Geometry check sheet. Reference: the model listing, model coordinates, mm. A direction names the side the tool comes from. Give positions to 0.01 mm unless a question says otherwise; leave off trailing zeros. Loops run counter-clockwise (first coordinate to the right, second up) from the corner with the lowest first, then second, coordinate; pieces in that order, holes last. Notation, with made-up numbers: (-38, -33.5) - (2, -33.5) arc R21 cw to (2, 0.5) - close; hole circle Ø1 at (71.25, -31). An arc over 180 degrees is marked (long way). Use a Markdown table: item, result. Add a question column.
1. Set-up check for faces 1 (the flat face through (0, -21.59, 0)), 2 (the flat face through (-1, 0, -20.32)), 3 (the flat face through (20.32, 0, 23)), 4 (the flat face through (-1.905, 0, 23)): record each of +Z, -Z, +X, -X, +Y, -Y from which the full face is reachable in a straight line by a thin tool's end or side.
2. Cross-section at A-A on x = 4. Enter the section's corners in (y, z), and give its area (3 significant figures).
3. Draft check along Z on faces 5 (the flat face through (0, -25.4, 0)), 6 (the flat face through (0, 0, -25.4)), 7 (the flat face through (1, 0, 20.32)). Enter one of: pulls with the +Z half, pulls with the -Z half, needs draft (parallel to the pull), parting line crosses it, or undercut.
4. Cross-section at D-D on z = -22. Enter the section's corners in (x, y) (3 decimals), and give its area (3 significant figures).
5. Material ranges on L1, parallel to Y at x = -13.5, z = 2; L2, parallel to X at y = -17.5, z = -23 (3 decimals); L3, parallel to Z at x = 1.5, y = 5, recorded low to high.
6. Cross-section at B-B on y = -11.5. Count the separate pieces of the cut face and the enclosed holes in it, and give its area (3 significant figures).
7. Cross-section at C-C on z = 17. Enter the section's corners in (x, y).
8. Depth check by flat-ended pin: P1, Ø6, axis at x = 5.5, y = 4.5, coming from the +Z side. Enter the tip coordinate at first touch or a pass-through.
from build123d import *

# Parameters (mm, degrees)
SKETCH1_W           = 5.08
SKETCH1_H           = 5.08
BOSS_EXTRUDE1_DEPTH = 21.59
LPATTERN2_COUNT     = 3
LPATTERN2_PITCH     = 22.86
LPATTERN3_COUNT     = 2
LPATTERN3_PITCH     = 23.495
LPATTERN4_COUNT     = 2
LPATTERN4_PITCH     = 23.495
SKETCH2_W           = 50.8
SKETCH2_H           = 50.8
BOSS_EXTRUDE3_DEPTH = 3.81
SKETCH3_W           = 50.8
SKETCH3_H           = 50.8
BOSS_EXTRUDE4_DEPTH = 3.81


with BuildPart() as part:
    # Sketch1 → Boss-Extrude1 (new body, symmetric)
    with BuildSketch(Plane(origin=(0, 0, 0), x_dir=(1, 0, 0), z_dir=(0, 1, 0))):
        with Locations((-22.86, -22.86)):
            Rectangle(SKETCH1_W, SKETCH1_H)
    extrude(amount=BOSS_EXTRUDE1_DEPTH, both=True)


with BuildPart() as lpattern2_1:
    # LPattern2: pattern copy
    add(part.part.moved(Location(Vector(0, 0, -1) * (1 * LPATTERN2_PITCH))))


with BuildPart() as lpattern2_2:
    # LPattern2: pattern copy
    add(part.part.moved(Location(Vector(0, 0, -1) * (2 * LPATTERN2_PITCH))))


with BuildPart() as body_4:
    # Mirror1: mirrored copy
    add(lpattern2_2.part.mirror(Plane(origin=(0, 0, 0), x_dir=(0, 0, 1), z_dir=(1, 0, 0))))


with BuildPart() as body_5:
    # Mirror1 2: mirrored copy
    add(lpattern2_1.part.mirror(Plane(origin=(0, 0, 0), x_dir=(0, 0, 1), z_dir=(1, 0, 0))))


with BuildPart() as body_6:
    # Mirror1 3: mirrored copy
    add(part.part.mirror(Plane(origin=(0, 0, 0), x_dir=(0, 0, 1), z_dir=(1, 0, 0))))


with BuildPart() as lpattern3_1:
    # LPattern3: pattern copy
    add(part.part.moved(Location(Vector(1, 0, 0) * (1 * LPATTERN3_PITCH))))


with BuildPart() as lpattern4_1:
    # LPattern4: pattern copy
    add(body_4.part.moved(Location(Vector(-1, 0, 0) * (1 * LPATTERN4_PITCH))))


with BuildPart() as part_1:
    add(part.part)

    add(lpattern2_1.part)  # Boss-Extrude3 merges LPattern2_1

    add(lpattern2_2.part)  # Boss-Extrude3 merges LPattern2_2

    add(body_4.part)  # Boss-Extrude3 merges body 4

    add(body_5.part)  # Boss-Extrude3 merges body 5

    add(body_6.part)  # Boss-Extrude3 merges body 6

    add(lpattern3_1.part)  # Boss-Extrude3 merges LPattern3_1

    add(lpattern4_1.part)  # Boss-Extrude3 merges LPattern4_1
    # Sketch2 → Boss-Extrude3 (add)
    with BuildSketch(Plane(origin=(0, 21.59, 0), x_dir=(1, 0, 0), z_dir=(0, 1, 0))):
        Rectangle(SKETCH2_W, SKETCH2_H)
    extrude(amount=BOSS_EXTRUDE3_DEPTH)

    # Sketch3 → Boss-Extrude4 (add)
    with BuildSketch(Plane.XZ.offset(21.59)):
        Rectangle(SKETCH3_W, SKETCH3_H)
    extrude(amount=BOSS_EXTRUDE4_DEPTH)


solid = part_1.part
Values found:
| question | item | result |
|---|---|---|
| 1 | face 1 | none |
| 1 | face 2 | +X, -X |
| 1 | face 3 | +Z, -Z |
| 1 | face 4 | +Z |
| 2 | outline | (-25.4, -25.4) - (-21.59, -25.4) - (-21.59, 25.4) - (-25.4, 25.4) - close; (21.59, -25.4) - (25.4, -25.4) - (25.4, 25.4) - (21.59, 25.4) - close |
| 2 | area | 387 mm2 |
| 3 | face 5 | needs draft |
| 3 | face 6 | pulls with the -Z half |
| 3 | face 7 | undercut |
| 4 | outline | (-25.4, -25.4) - (25.4, -25.4) - (25.4, 25.4) - (-25.4, 25.4) - close; hole (-20.32, -21.59) - (-3.175, -21.59) - (-3.175, 21.59) - (-20.32, 21.59) - close; hole (1.905, -21.59) - (20.32, -21.59) - (20.32, 21.59) - (1.905, 21.59) - close |
| 4 | area | 1,050 mm2 |
| 5 | L1 | y = -25.4 to -21.59, 21.59 to 25.4 |
| 5 | L2 | x = -25.4 to -20.32, -3.175 to 1.905, 20.32 to 25.4 |
| 5 | L3 | z = -25.4 to -20.32, 20.32 to 25.4 |
| 6 | separate pieces | 8 |
| 6 | enclosed holes | 0 |
| 6 | area | 206 mm2 |
| 7 | outline | (-25.4, -25.4) - (25.4, -25.4) - (25.4, -21.59) - (-25.4, -21.59) - close; (-25.4, 21.59) - (25.4, 21.59) - (25.4, 25.4) - (-25.4, 25.4) - close |
| 8 | P1 | stops at z = 25.4 |
